Could you check a few things on this model? Use its own coordinates, in mm. Coordinates: 2 decimals unless noted, no trailing zeros. Loops run counter-clockwise (first coordinate to the right, second up) from the corner with the lowest first, then second, coordinate; pieces in that order, holes last. Notation, with made-up numbers: (-7, 64.5) -> (17, 64.5) arc R19 cw to (17, 93.5) -> close; hole circle Ø1 at (-36.75, -5). An arc over 180 degrees is marked (long way). One line per question, with ' | ' between items.
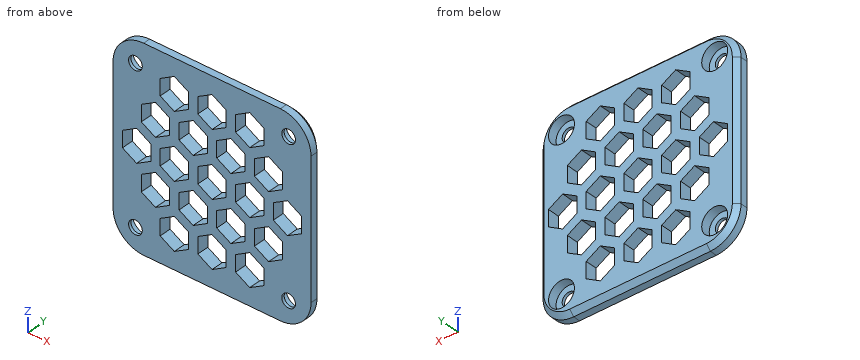
```python
from build123d import *

# Parameters (mm, degrees)
BOSS_EXTRUDE1_DEPTH                                  = 2.5
CBORE_FOR_M2_5_HEX_SOCKET_HEAD_CAP_SCREW_D           = 2.9
CBORE_FOR_M2_5_HEX_SOCKET_HEAD_CAP_SCREW_CBORE_D     = 5.5
CBORE_FOR_M2_5_HEX_SOCKET_HEAD_CAP_SCREW_CBORE_DEPTH = 1.9
FILL_PATTERN2_DEPTH                                  = 2.5
CHAMFER1_SIZE                                        = 1


# Read off the part's stored shape, not the designer's step: Fill Pattern2
with BuildPart() as part:
    # Sketch1 → Boss-Extrude1 (new body)
    with BuildSketch(Plane(origin=(0, 0, 0), x_dir=(1, 0, 0), z_dir=(0, 1, 0))):
        with BuildLine():
            Line((6.5, 0), (35.5, 0))
            ThreePointArc((35.5, 0), (40.096194078, -1.903805922), (42, -6.5))
            Line((42, -6.5), (42, -35.5))
            ThreePointArc((42, -35.5), (40.096194078, -40.096194078), (35.5, -42))
            Line((35.5, -42), (6.5, -42))
            ThreePointArc((6.5, -42), (1.903805922, -40.096194078), (0, -35.5))
            Line((0, -35.5), (0, -6.5))
            ThreePointArc((0, -6.5), (1.903805922, -1.903805922), (6.5, 0))
        make_face()
    extrude(amount=BOSS_EXTRUDE1_DEPTH)

    # CBORE for M2.5 Hex Socket Head Cap Screw1 (through all)
    with Locations(Plane(origin=(0, 2.5, 0), x_dir=(1, 0, 0), z_dir=(0, 1, 0))):
        with Locations((4.75, -37.25), (4.75, -4.75), (37.25, -4.75), (37.25, -37.25)):
            CounterBoreHole(CBORE_FOR_M2_5_HEX_SOCKET_HEAD_CAP_SCREW_D / 2, CBORE_FOR_M2_5_HEX_SOCKET_HEAD_CAP_SCREW_CBORE_D / 2, CBORE_FOR_M2_5_HEX_SOCKET_HEAD_CAP_SCREW_CBORE_DEPTH)

    # Fill Pattern2 outline → Fill Pattern2 (cut)
    with BuildSketch(Plane(origin=(0, 0, 0), x_dir=(1, 0, 0), z_dir=(0, 1, 0))):
        Polygon((8, -19.267949192), (5, -17.535898385), (2, -19.267949192), (2, -22.732050808), (5, -24.464101615), (8, -22.732050808), align=None)
        Polygon((20, -26.196152423), (17, -24.464101615), (14, -26.196152423), (14, -29.660254038), (17, -31.392304845), (20, -29.660254038), align=None)
        Polygon((32, -33.124355653), (29, -31.392304845), (26, -33.124355653), (26, -36.588457268), (29, -38.320508076), (32, -36.588457268), align=None)
        Polygon((29, -3.679491924), (26, -5.411542732), (26, -8.875644347), (29, -10.607695155), (32, -8.875644347), (32, -5.411542732), align=None)
        Polygon((17, -10.607695155), (14, -12.339745962), (14, -15.803847577), (17, -17.535898385), (20, -15.803847577), (20, -12.339745962), align=None)
        Polygon((36, -12.339745962), (33, -10.607695155), (30, -12.339745962), (30, -15.803847577), (33, -17.535898385), (36, -15.803847577), align=None)
        Polygon((24, -5.411542732), (21, -3.679491924), (18, -5.411542732), (18, -8.875644347), (21, -10.607695155), (24, -8.875644347), align=None)
        Polygon((9, -24.464101615), (6, -26.196152423), (6, -29.660254038), (9, -31.392304845), (12, -29.660254038), (12, -26.196152423), align=None)
        Polygon((21, -17.535898385), (18, -19.267949192), (18, -22.732050808), (21, -24.464101615), (24, -22.732050808), (24, -19.267949192), align=None)
        Polygon((30, -26.196152423), (30, -29.660254038), (33, -31.392304845), (36, -29.660254038), (36, -26.196152423), (33, -24.464101615), align=None)
        Polygon((26, -19.267949192), (26, -22.732050808), (29, -24.464101615), (32, -22.732050808), (32, -19.267949192), (29, -17.535898385), align=None)
        Polygon((16, -19.267949192), (13, -17.535898385), (10, -19.267949192), (10, -22.732050808), (13, -24.464101615), (16, -22.732050808), align=None)
        Polygon((28, -26.196152423), (25, -24.464101615), (22, -26.196152423), (22, -29.660254038), (25, -31.392304845), (28, -29.660254038), align=None)
        Polygon((25, -10.607695155), (22, -12.339745962), (22, -15.803847577), (25, -17.535898385), (28, -15.803847577), (28, -12.339745962), align=None)
        Polygon((10, -33.124355653), (10, -36.588457268), (13, -38.320508076), (16, -36.588457268), (16, -33.124355653), (13, -31.392304845), align=None)
        Polygon((10, -5.411542732), (10, -8.875644347), (13, -10.607695155), (16, -8.875644347), (16, -5.411542732), (13, -3.679491924), align=None)
        Polygon((12, -12.339745962), (9, -10.607695155), (6, -12.339745962), (6, -15.803847577), (9, -17.535898385), (12, -15.803847577), align=None)
        Polygon((37, -17.535898385), (34, -19.267949192), (34, -22.732050808), (37, -24.464101615), (40, -22.732050808), (40, -19.267949192), align=None)
        Polygon((24, -33.124355653), (21, -31.392304845), (18, -33.124355653), (18, -36.588457268), (21, -38.320508076), (24, -36.588457268), align=None)
    extrude(amount=FILL_PATTERN2_DEPTH, mode=Mode.SUBTRACT)

    # Chamfer1
    chamfer1_edges = [part.edges().sort_by_distance(p)[0] for p in [
        (40.096194078, 2.5, 1.903805922),
        (21, 2.5, 0),
        (1.903805922, 2.5, 1.903805922),
        (0, 2.5, 21),
        (1.903805922, 2.5, 40.096194078),
        (21, 2.5, 42),
        (40.096194078, 2.5, 40.096194078),
        (42, 2.5, 21),
    ]]
    chamfer(chamfer1_edges, length=CHAMFER1_SIZE)


solid = part.part
```
Q1. Imagine slicing it at A-A on z = 23.5. Write out the boundary of the cut face in (x, y).
Values follow:
outline: (0, 0) -> (3.33, 0) -> (3.33, 2.5) -> (1, 2.5) -> (0, 1.5) -> close; (6.67, 0) -> (11.33, 0) -> (11.33, 2.5) -> (6.67, 2.5) -> close; (14.67, 0) -> (19.33, 0) -> (19.33, 2.5) -> (14.67, 2.5) -> close; (22.67, 0) -> (27.33, 0) -> (27.33, 2.5) -> (22.67, 2.5) -> close; (30.67, 0) -> (35.33, 0) -> (35.33, 2.5) -> (30.67, 2.5) -> close; (38.67, 0) -> (42, 0) -> (42, 1.5) -> (41, 2.5) -> (38.67, 2.5) -> close
Q2. Please list where these lines run through material, in increasing order: L1, parallel to Z at x = 29, y = 1.4; L2, parallel to X at y = 1.05, z = 34; L3, parallel to Z at x = 9, y = 1.45. Write a range as [from, to].
Values follow:
L1: z = [0, 3.68], [10.61, 17.54], [24.46, 31.39], [38.32, 42] | L2: x = [0, 10], [16, 18], [24, 26], [32, 42] | L3: z = [0, 10.61], [17.54, 24.46], [31.39, 42]
Q3. Imagine slicing it at B-B on z = 7. Write out the boundary of the cut face in (x, y).
Values follow:
outline: (0, 0) -> (10, 0) -> (10, 2.5) -> (6.33, 2.5) -> (6.33, 0.6) -> (3.17, 0.6) -> (3.17, 2.5) -> (1, 2.5) -> (0, 1.5) -> close; (16, 0) -> (18, 0) -> (18, 2.5) -> (16, 2.5) -> close; (24, 0) -> (26, 0) -> (26, 2.5) -> (24, 2.5) -> close; (32, 0) -> (42, 0) -> (42, 1.5) -> (41, 2.5) -> (38.83, 2.5) -> (38.83, 0.6) -> (35.67, 0.6) -> (35.67, 2.5) -> (32, 2.5) -> close
Q4. Imagine slicing it at D-D on x = 22.5. Write out the boundary of the cut face in (y, z), plus the area to 3 significant figures.
Values follow:
outline: (0, 0) -> (1.5, 0) -> (2.5, 1) -> (2.5, 4.55) -> (0, 4.55) -> close; (0, 9.74) -> (2.5, 9.74) -> (2.5, 12.05) -> (0, 12.05) -> close; (0, 16.09) -> (2.5, 16.09) -> (2.5, 18.4) -> (0, 18.4) -> close; (0, 23.6) -> (2.5, 23.6) -> (2.5, 25.91) -> (0, 25.91) -> close; (0, 29.95) -> (2.5, 29.95) -> (2.5, 32.26) -> (0, 32.26) -> close; (0, 37.45) -> (2.5, 37.45) -> (2.5, 41) -> (1.5, 42) -> (0, 42) -> close | area: 44.8 mm2
Q5. Imagine slicing it at C-C on x = 29.5. Write out the boundary of the cut face in (y, z), plus the area to 3 significant figures.
Values follow:
outline: (0, 0) -> (1.5, 0) -> (2.5, 1) -> (2.5, 3.97) -> (0, 3.97) -> close; (0, 10.32) -> (2.5, 10.32) -> (2.5, 17.82) -> (0, 17.82) -> close; (0, 24.18) -> (2.5, 24.18) -> (2.5, 31.68) -> (0, 31.68) -> close; (0, 38.03) -> (2.5, 38.03) -> (2.5, 41) -> (1.5, 42) -> (0, 42) -> close | area: 56.4 mm2
